Drawing for the job (mm, zero at the part's lowest x, y, z). A direction names the side the tool comes from. Coordinates: 2 decimals unless noted, no trailing zeros. Loops run counter-clockwise (first coordinate to the right, second up) from the corner with the lowest first, then second, coordinate; pieces in that order, holes last. Notation, with made-up numbers: (-40, -7) -> (-24, -7) arc R30 ccw to (-24, 21) -> close; hole circle Ø1 at (-0.5, 13.5). An arc over 180 degrees is marked (long way). Write each question's results on one line, items separated by ' | '.
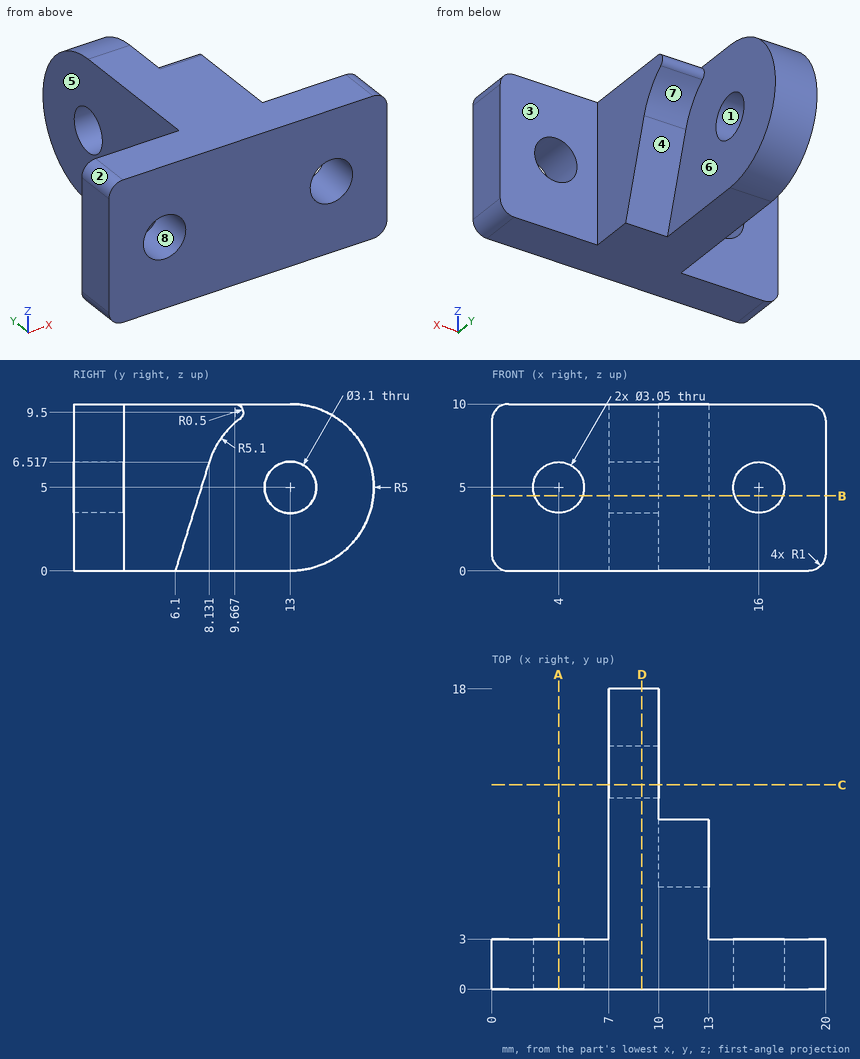
1) Drill centre lines: L1, parallel to X at y = 1.2, z = 5 (1 decimal); L2, parallel to Z at x = 8.8, y = 13; L3, parallel to Y at x = 8.75, z = 5. Where is each one in solid material? Low to high. Write a range as from..to.
Outcome:
L1: x = 0..2.5, 5.5..14.5, 17.5..20 | L2: z = 0..3.45, 6.55..10 | L3: y = 0..11.45, 14.55..18
2) Slice it at A-A (x = 4). Write the cut outline in (y, z) (1 decimal).
Outcome:
outline: (0, 0) -> (3, 0) -> (3, 3.5) -> (0, 3.5) -> close; (0, 6.5) -> (3, 6.5) -> (3, 10) -> (0, 10) -> close
3) Which spindle directions (+Z, -Z, +X, -X, +Y, -Y) get a long thin tool onto all of the face, cutting with end or side? Do the marked faces 1, 2, 3, 4 and 5. Say none if no direction does.
Outcome:
face 1: +X, -X | face 2: +Z, -X, +Y, -Y | face 3: +Z, -Z, +X, +Y | face 4: -Z, +X, +Y | face 5: +Z, -Z, -X, +Y
4) Pin check, flat tips, straight feed: pin 1 (2 mm diameter, centred on x = 17.5, z = 5.5, fed in from +Y); pin 2 (6 mm diameter, centred on y = 11, z = 2.5, fed in from +X); pin 3 (2 mm diameter, centred on y = 5.5, z = 3, fed in from +X); pin 4 (2.5 mm diameter, centred on x = 4, z = 5, fed in from -Y). Stop position of each tip, or through.
Outcome:
pin 1: stops at y = 3 | pin 2: stops at x = 10 | pin 3: stops at x = 13 | pin 4: passes through
5) Two-plate mould, pull along X, no slides. Class the marked faces 6, 7 and 8: pulls with the +X half, pulls with the -X half, needs draft (parallel to the pull), parting line crosses it, or undercut.
Outcome:
face 6: pulls with the +X half | face 7: needs draft | face 8: undercut
6) Slice it at C-C (y = 12.25). Write the cut outline in (x, z).
Outcome:
outline: (7, 0) -> (10, 0) -> (10, 3.64) -> (7, 3.64) -> close; (7, 6.36) -> (10, 6.36) -> (10, 10) -> (7, 10) -> close
7) Slice it at B-B (z = 4.5). Write the cut outline in (x, y) (1 decimal).
Outcome:
outline: (0, 0) -> (2.6, 0) -> (2.6, 3) -> (0, 3) -> close; (5.4, 0) -> (14.6, 0) -> (14.6, 3) -> (13, 3) -> (13, 7.5) -> (10, 7.5) -> (10, 11.5) -> (7, 11.5) -> (7, 3) -> (5.4, 3) -> close; (7, 14.5) -> (10, 14.5) -> (10, 18) -> (7, 18) -> close; (17.4, 0) -> (20, 0) -> (20, 3) -> (17.4, 3) -> close
8) Slice it at D-D (x = 9). Write the cut outline in (y, z).
Outcome:
outline: (0, 0) -> (13, 0) arc R5 ccw to (13, 10) -> (0, 10) -> close; hole circle Ø3.1 at (13, 5)
